Here's how the part is built. I have some questions about the finished solid (model axes, mm). A direction names the side the tool comes from. Round coordinates to 2 decimals unless told otherwise and drop trailing zeros. Write each loop counter-clockwise with the first axis right and the second up, starting at its lowest first coordinate (ties: lowest second). Pieces come first, ordered by that corner, then holes. Notation, with made-up numbers: (-37.75, 3.25) -> (-21.75, 3.25) arc R19 cw to (-21.75, 39.25) -> close; hole circle Ø11 at (69.25, 33). An arc over 180 degrees is marked (long way). Answer as CSV lines item,"result".
```python
from build123d import *

# Parameters (mm, degrees)
PAD_DEPTH         = 5.5
SKETCH001_W       = 6
SKETCH001_H       = 10
PAD001_DEPTH      = 4.5
PAD001_DEPTH_BACK = 10.5
SKETCH002_R       = 2.25
POCKET_DEPTH      = 5


with BuildPart() as part:
    # Sketch → Pad (new body)
    with BuildSketch(Plane.XY):
        Polygon((-12.6, 18), (-12.6, 0), (0, 0), (0, -10), (6, -10), (6, 5.4), (-6.6, 18), align=None)
    extrude(amount=PAD_DEPTH)

    # Sketch001 (on Face9 of Pad) → Pad001 (join, two sides)
    with BuildSketch(Plane.XY.offset(5.5)) as pad001_sk:
        with Locations((3, -5)):
            Rectangle(SKETCH001_W, SKETCH001_H)
    extrude(amount=PAD001_DEPTH)
    extrude(pad001_sk.sketch, amount=-PAD001_DEPTH_BACK)

    # Sketch002 (on Face4 of Pad001) → Pocket (cut)
    with BuildSketch(Plane(origin=(0, 0, 0), x_dir=(1, 0, 0), z_dir=(0, 0, -1))):
        with Locations((-9.6, -7.4)):
            Circle(SKETCH002_R)
        with Locations((-9.6, -12.4)):
            Circle(SKETCH002_R)
    extrude(amount=-POCKET_DEPTH, mode=Mode.SUBTRACT)


solid = part.part
```
1. If I drill on line 1 (Y direction, x = -9.6, z = 2.05); line 2 (X direction, y = -8.25, z = 3.5); line 3 (Z direction, x = -7.5, y = 15), over which ranges is the centre line in solid material (lowest first)?
Numbers:
line 1,"y = 0 to 5.15, 9.65 to 10.15, 14.65 to 18"
line 2,"x = 0 to 6"
line 3,"z = 0 to 5.5"
2. Suppose I cut it at B-B on y = 12.4. Please give me the cut outline in (x, z), and give its area (3 significant figures).
Numbers:
outline,"(-12.6, 0) -> (-11.85, 0) -> (-11.85, 5) -> (-7.35, 5) -> (-7.35, 0) -> (-1, 0) -> (-1, 5.5) -> (-12.6, 5.5) -> close"
area,"41.3 mm^2"
3. On a 3-axis mill with a long thin cutter (end or side, diameter ignored), from which of +Z, -Z, +X, -X, +Y, -Y can I reach the whole of each face in a straight line? I mean faces 1 (the face through (-6, 0, 3)), 2 (the face through (3, 0, -2)), 3 (the face through (3, 0, 8)), 4 (the face through (-10, 7, 5)). Say none if no direction works.
Numbers:
face 1,"+Z, -Z, -X, -Y"
face 2,"-Z, +X, -X, +Y"
face 3,"+Z, +X, -X, +Y"
face 4,"-Z"
4. Suppose I cut it at D-D on z = 6. Please give me the cut outline in (x, y), and give its area (3 significant figures).
Numbers:
outline,"(0, -10) -> (6, -10) -> (6, 0) -> (0, 0) -> close"
area,"60.0 mm^2"
5. Suppose I cut it at A-A on z = 0.5. Please give me the cut outline in (x, y), and give its area (3 significant figures).
Numbers:
outline,"(-12.6, 0) -> (0, 0) -> (0, -10) -> (6, -10) -> (6, 5.4) -> (-6.6, 18) -> (-12.6, 18) -> close; hole circle Ø4.5 at (-9.6, 7.4); hole circle Ø4.5 at (-9.6, 12.4)"
area,"284 mm^2"
6. For pin 1 Ø5 at (x, y) = (-9.6, 7.4) entering from +Z; pin 2 Ø3 at (x, z) = (-3, 3.5) entering from -Y; pin 3 Ø2.5 at (x, z) = (1.5, -2) entering from +Y, each with a flat end and sliding along its axis, tell me the tip position at first contact or that it passes through.
Numbers:
pin 1,"stops at z = 5.5"
pin 2,"stops at y = 0"
pin 3,"stops at y = 0"
7. Suppose I cut it at C-C on x = 4.75. Please give me the cut outline in (y, z), and give its area (3 significant figures).
Numbers:
outline,"(-10, -5) -> (0, -5) -> (0, 0) -> (6.65, 0) -> (6.65, 5.5) -> (0, 5.5) -> (0, 10) -> (-10, 10) -> close"
area,"187 mm^2"
8. If we mould it in two halves opening along X, with no side actions, what happens to faces 5 (the face through (-10, 12, 5)), 6 (the face through (0, -5, 3)), 7 (the face through (3, -5, 10))? For each: released by +X, released by -X, zero draft, split by the parting line, or undercut.
Numbers:
face 5,"undercut"
face 6,"released by -X"
face 7,"zero draft"
